Source: CAD feature listing. Evaluate the final solid. Frame: model axes, mm. Face numbers are marked on the shaded views. A direction names the side the tool comes from. Round coordinates to 2 decimals unless told otherwise and drop trailing zeros. Loops run counter-clockwise (first coordinate to the right, second up) from the corner with the lowest first, then second, coordinate; pieces in that order, holes last.
Item 1: Section query D-D on z = 2.25. Return loops of the section in (x, y), then the cut area to 3 significant figures.
Item 2: Access query for the marked faces 4, 5 and 6. Directions: +Z, -Z, +X, -X, +Y, -Y. A direction counts if a zero-diameter tool reaches every point of the face in a straight line with its end or side. Return the directions, or none.
Item 3: Pull-direction query (Y, two-part tool) for the marked faces 1, 2 and 3; classes: released by +Y, released by -Y, zero draft, split by the parting line, or undercut.
Item 4: First-contact query: P1, Ø5.5, axis at x = 0, z = -21.5, coming from the +Y side; P2, Ø1.5, axis at x = 0, z = -21, coming from the -Y side; P3, Ø6, axis at x = -2.5, y = 7, coming from the +Z side; P4, Ø4, axis at x = 2, y = -2.5, coming from the +Z side. Flat tips, straight axial feed; report the tip coordinate or a pass-through.
Item 5: Section query A-A on z = -23. Return loops of the section in (x, y), then the cut area to 3 significant figures.
Item 6: Ray query, L1, parallel to Y at x = -0.5, z = -21.5; L2, parallel to Z at x = -2, y = -3; L3, parallel to Y at x = -0.75, z = 2.25. Return the intervals inside material, ascending.
Item 7: Section query C-C on y = 0. Return loops of the section in (x, z), then the cut area to 3 significant figures.
Item 8: Section query B-B on x = -2. Return loops of the section in (y, z), then the cut area to 3 significant figures.
```python
from build123d import *

# Parameters (mm, degrees)
SKETCH1_W                      = 18.7
SKETCH1_H                      = 46
BOSS_EXTRUDE1_DEPTH            = 10
SKETCH2_W                      = 18
SKETCH2_H                      = 7.5
CUT_EXTRUDE1_DEPTH             = 31.870698081
SKETCH3_W                      = 18
SKETCH3_H                      = 7.5
CUT_EXTRUDE2_DEPTH             = 31.870698081
SKETCH4_W                      = 5
SKETCH4_H                      = 0.5
BOSS_EXTRUDE2_DEPTH            = 7
SKETCH5_W                      = 5
SKETCH5_H                      = 0.5
BOSS_EXTRUDE3_DEPTH            = 7
SKETCH6_W                      = 1.45
SKETCH6_H                      = 3.8
F_2_5_2_5_DIAMETER_HOLE1_D     = 2.5
F_2_5_2_5_DIAMETER_HOLE1_DEPTH = 25.7
FILLET1_R                      = 0.5
CUT_EXTRUDE3_DEPTH             = 35.336569427
CUT_EXTRUDE3_DEPTH_BACK        = 35.336569427


with BuildPart() as part:
    # Sketch1 → Boss-Extrude1 (new body)
    with BuildSketch(Plane(origin=(5, 0, 0), x_dir=(0, 0, -1), z_dir=(1, 0, 0))):
        with Locations((8.65, 0)):
            Rectangle(SKETCH1_W, SKETCH1_H)
    extrude(amount=-BOSS_EXTRUDE1_DEPTH)

    # Sketch2 → Cut-Extrude1 (cut, through all)
    with BuildSketch(Plane.ZY.offset(5)):
        with Locations((-9, -19.25)):
            Rectangle(SKETCH2_W, SKETCH2_H)
    extrude(amount=-CUT_EXTRUDE1_DEPTH, mode=Mode.SUBTRACT)

    # Sketch3 → Cut-Extrude2 (cut, through all)
    with BuildSketch(Plane.ZY.offset(5)):
        with Locations((-9, 19.25)):
            Rectangle(SKETCH3_W, SKETCH3_H)
    extrude(amount=-CUT_EXTRUDE2_DEPTH, mode=Mode.SUBTRACT)

    # Sketch4 → Boss-Extrude2 (add)
    with BuildSketch(Plane(origin=(0, 0, -18), x_dir=(-1, 0, 0), z_dir=(0, 0, -1))):
        with Locations((0, -7.25)):
            Rectangle(SKETCH4_W, SKETCH4_H)
    extrude(amount=BOSS_EXTRUDE2_DEPTH)

    # Sketch5 → Boss-Extrude3 (add)
    with BuildSketch(Plane(origin=(0, 0, -18), x_dir=(-1, 0, 0), z_dir=(0, 0, -1))):
        with Locations((0, 13.75)):
            Rectangle(SKETCH5_W, SKETCH5_H)
    extrude(amount=BOSS_EXTRUDE3_DEPTH)

    # Sketch6 → Revolve1 (revolve)
    with BuildSketch(Plane.XZ, mode=Mode.PRIVATE) as revolve1_sk:
        with Locations((0.725, 2.6)):
            Rectangle(SKETCH6_W, SKETCH6_H)
    revolve(revolve1_sk.sketch.rotate(Axis((0, 0, 4.5), (0, 0, -1)), 180), axis=Axis((0, 0, 4.5), (0, 0, -1)))

    # Ø2.5 (2.5) Diameter Hole1
    with Locations(Plane.XY.offset(0.7)):
        with Locations((0, -21), (0, 21)):
            Hole(F_2_5_2_5_DIAMETER_HOLE1_D / 2, depth=F_2_5_2_5_DIAMETER_HOLE1_DEPTH)

    # Fillet1
    fillet1_edges = [part.edges().sort_by_distance(p)[0] for p in [
        (5, 23, 0.35),
        (-5, 23, 0.35),
        (-5, -23, 0.35),
        (5, -23, 0.35),
    ]]
    fillet(fillet1_edges, radius=FILLET1_R)

    # Sketch9 → Cut-Extrude3 (cut, two sides: drawn at the far end of the back side and taken through both)
    with BuildSketch(Plane(origin=(0, 0, 0), x_dir=(-1, 0, 0), z_dir=(0, 0, -1)).offset(-CUT_EXTRUDE3_DEPTH_BACK)):
        with BuildLine():
            Line((4.5, 23), (-4.5, 23))
            ThreePointArc((-4.5, 23), (-4.853553391, 22.853553391), (-5, 22.5))
            Line((-5, 22.5), (-5, 15.5))
            Line((-5, 15.5), (5, 15.5))
            Line((5, 15.5), (5, 22.5))
            ThreePointArc((5, 22.5), (4.853553391, 22.853553391), (4.5, 23))
        make_face()
        with BuildLine():
            Line((-4.5, -23), (4.5, -23))
            ThreePointArc((4.5, -23), (4.853553391, -22.853553391), (5, -22.5))
            Line((5, -22.5), (5, -15.5))
            Line((5, -15.5), (-5, -15.5))
            Line((-5, -15.5), (-5, -22.5))
            ThreePointArc((-5, -22.5), (-4.853553391, -22.853553391), (-4.5, -23))
        make_face()
    extrude(amount=CUT_EXTRUDE3_DEPTH + CUT_EXTRUDE3_DEPTH_BACK, mode=Mode.SUBTRACT)


solid = part.part
```
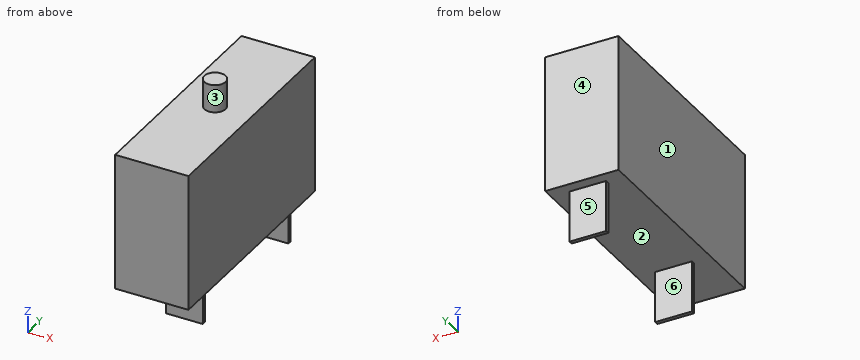
Data:
1. outline: circle Ø2.9 at (0, 0)
1. area: 6.61 mm2
2. face 4: +Z, -Z, +X, -X, +Y
2. face 5: -Z, +X, -X, +Y
2. face 6: -Z, +X, -X
3. face 1: zero draft
3. face 2: undercut
3. face 3: split by the parting line
4. P1: stops at y = 14
4. P2: stops at y = -7.5
4. P3: stops at z = 0.7
4. P4: stops at z = 4.5
5. outline: (-2.5, -7.5) - (2.5, -7.5) - (2.5, -7) - (-2.5, -7) - close; (-2.5, 13.5) - (2.5, 13.5) - (2.5, 14) - (-2.5, 14) - close
5. area: 5.00 mm2
6. L1: y = -7.5 to -7, 13.5 to 14
6. L2: z = -18 to 0.7
6. L3: y = -1.24 to 1.24
7. outline: (-5, -18) - (5, -18) - (5, 0.7) - (1.45, 0.7) - (1.45, 4.5) - (-1.45, 4.5) - (-1.45, 0.7) - (-5, 0.7) - close
7. area: 198 mm2
8. outline: (-15.5, -18) - (-7.5, -18) - (-7.5, -25) - (-7, -25) - (-7, -18) - (13.5, -18) - (13.5, -25) - (14, -25) - (14, -18) - (15.5, -18) - (15.5, 0.7) - (-15.5, 0.7) - close
8. area: 587 mm2
